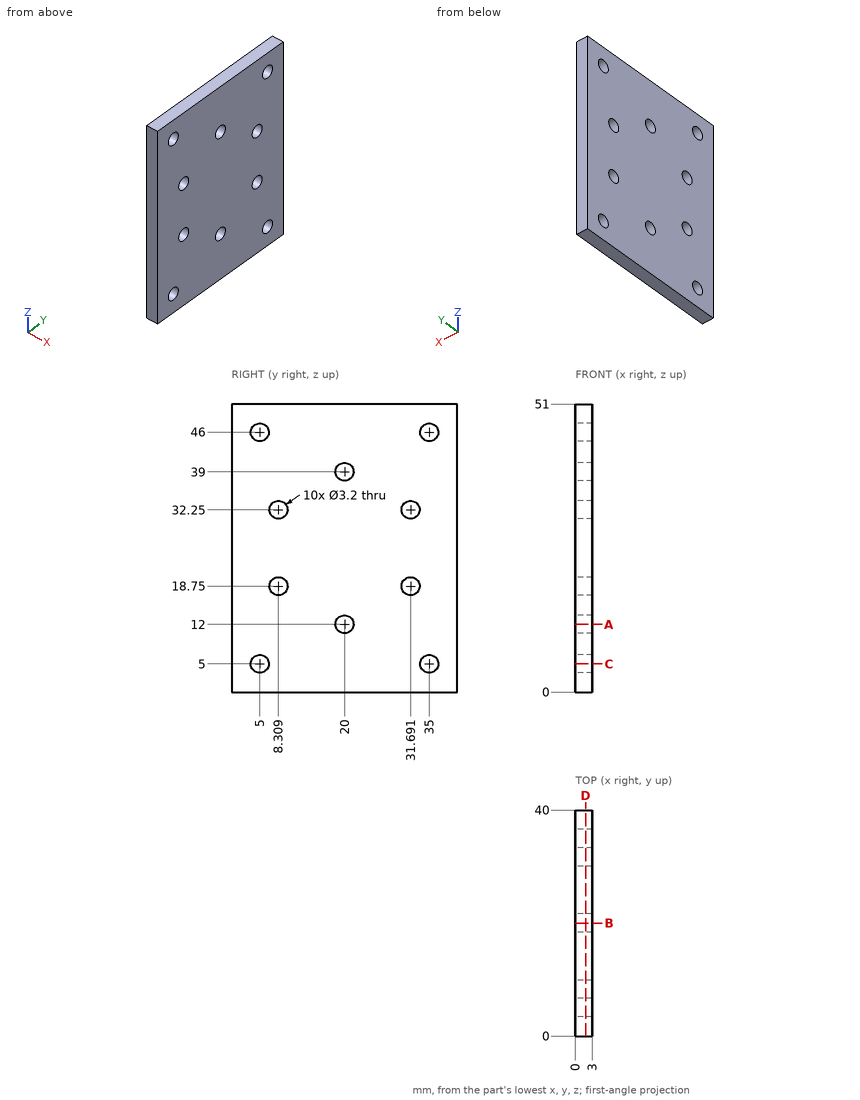
Drawing for the job (mm, zero at the part's lowest x, y, z). Coordinates: 2 decimals unless noted, no trailing zeros. Loops run counter-clockwise (first coordinate to the right, second up) from the corner with the lowest first, then second, coordinate; pieces in that order, holes last. Notation, with made-up numbers: (78, 69.25) - (105, 69.25) arc R22 cw to (105, 107.25) - close; hole circle Ø10 at (71, 62.25). An arc over 180 degrees is marked (long way). Return JSON: item names as keys, results as strings.
1. Probe L1, parallel to Y at x = 0.95, z = 5; L2, parallel to Y at x = 0.7, z = 32.25; L3, parallel to Y at x = 1.55, z = 12. List the from-to ranges inside material, lowest first. Write a range as from..to.
Result:
{"L1": "y = 0..3.4, 6.6..33.4, 36.6..40", "L2": "y = 0..6.71, 9.91..30.09, 33.29..40", "L3": "y = 0..18.4, 21.6..40"}
2. Drop a flat-ended pin along its axis: pin 1 (2.5 mm diameter, centred on y = 31.69, z = 32.25, fed in from +X). Give the stop position or say it passes through.
Result:
{"pin 1": "passes through"}
3. Band-saw the part on B-B (y = 20). Give the cut face in (x, z), and give its area (3 significant figures).
Result:
{"outline": "(0, 0) - (3, 0) - (3, 10.4) - (0, 10.4) - close; (0, 13.6) - (3, 13.6) - (3, 37.4) - (0, 37.4) - close; (0, 40.6) - (3, 40.6) - (3, 51) - (0, 51) - close", "area": "134 mm2"}
4. Band-saw the part on C-C (z = 5). Give the cut face in (x, y).
Result:
{"outline": "(0, 0) - (3, 0) - (3, 3.4) - (0, 3.4) - close; (0, 6.6) - (3, 6.6) - (3, 33.4) - (0, 33.4) - close; (0, 36.6) - (3, 36.6) - (3, 40) - (0, 40) - close"}
5. Band-saw the part on A-A (z = 12). Give the cut face in (x, y).
Result:
{"outline": "(0, 0) - (3, 0) - (3, 18.4) - (0, 18.4) - close; (0, 21.6) - (3, 21.6) - (3, 40) - (0, 40) - close"}
6. Band-saw the part on D-D (x = 1.8). State how many separate pieces and enclosed holes the cut face has, and give its area (3 significant figures).
Result:
{"separate pieces": "1", "enclosed holes": "10", "area": "1,960 mm2"}
